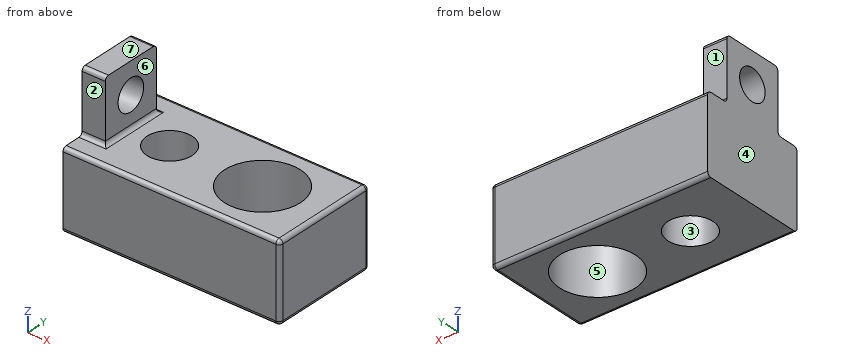
from build123d import *

# Parameters (mm, degrees)
SKETCH1_W           = 14
SKETCH1_H           = 7
BOSS_EXTRUDE1_DEPTH = 5
SKETCH2_R           = 2.45
SKETCH2_R_2         = 1.45
CUT_EXTRUDE1_DEPTH  = 10.287087811
SKETCH5_W           = 4
SKETCH5_H           = 4
BOSS_EXTRUDE3_DEPTH = 1.5
SKETCH9_R           = 1
CUT_EXTRUDE2_DEPTH  = 2
FILLET1_R           = 0.25


with BuildPart() as part:
    # Sketch1 → Boss-Extrude1 (new body)
    with BuildSketch(Plane.XY):
        Rectangle(SKETCH1_W, SKETCH1_H)
    extrude(amount=BOSS_EXTRUDE1_DEPTH)

    # Sketch2 → Cut-Extrude1 (cut, through all)
    with BuildSketch(Plane.XY):
        with Locations((3, 0)):
            Circle(SKETCH2_R)
        with Locations((-3, 0)):
            Circle(SKETCH2_R_2)
    extrude(amount=CUT_EXTRUDE1_DEPTH, mode=Mode.SUBTRACT)

    # Sketch5 → Boss-Extrude3 (add)
    with BuildSketch(Plane.ZY.offset(7)):
        with Locations((7, 0)):
            Rectangle(SKETCH5_W, SKETCH5_H)
    extrude(amount=-BOSS_EXTRUDE3_DEPTH)

    # Sketch9 → Cut-Extrude2 (cut)
    with BuildSketch(Plane(origin=(-5.5, 0, 0), x_dir=(0, 0, -1), z_dir=(1, 0, 0))):
        with Locations((-7, 0)):
            Circle(SKETCH9_R)
    extrude(amount=-CUT_EXTRUDE2_DEPTH, mode=Mode.SUBTRACT)

    # Fillet1
    fillet1_edges = [part.edges().sort_by_distance(p)[0] for p in [
        (7, 0, 5),
        (0, 3.5, 5),
        (-5.5, 0, 5),
        (-6.25, -2, 5),
        (-6.25, 2, 5),
        (-6.25, 2, 9),
        (-6.25, -2, 9),
        (0, 3.5, 0),
        (7, 0, 0),
        (0, -3.5, 0),
        (7, 3.5, 2.5),
        (7, -3.5, 2.5),
        (0, -3.5, 5),
    ]]
    fillet(fillet1_edges, radius=FILLET1_R)


solid = part.part
Can you work these out from the model? Positions are in its coordinate system, mm. Face numbers are marked on the shaded views. A direction names the side the tool comes from. Give positions to 0.01 mm unless a question says otherwise; leave off trailing zeros. Loops run counter-clockwise (first coordinate to the right, second up) from the corner with the lowest first, then second, coordinate; pieces in that order, holes last. Notation, with made-up numbers: M 7,88.5 L 15,88.5 A23 ccw 15,97.5 Z; hole C 51,49 d5. An arc over 180 degrees is marked long. One line per item, written item: value.
1) Imagine slicing it at B-B on x = -3. Write out the boundary of the cut face in (y, z).
Geometry check:
outline: M -3.5,0.25 A0.25 ccw -3.25,0 L -1.45,0 L -1.45,5 L -3.25,5 A0.25 ccw -3.5,4.75 Z; M 1.45,0 L 3.25,0 A0.25 ccw 3.5,0.25 L 3.5,4.75 A0.25 ccw 3.25,5 L 1.45,5 Z
2) On a 3-axis mill with a long thin cutter (end or side, diameter ignored), from which of +Z, -Z, +X, -X, +Y, -Y can I reach the whole of each face in a straight line? I mean the marked faces 1, 2 and 3. Say none if no direction works.
Geometry check:
face 1: +Z, +X, -X, +Y
face 2: +Z, +X, -X, -Y
face 3: +Z, -Z
3) I'm going to push flat-ended pins straight in: pin 1 (2 mm diameter, centred on x = 3.5, y = -2.5, fed in from +Z); pin 2 (1.1 mm diameter, centred on y = -1, z = 6.5, fed in from +X); pin 3 (1.2 mm diameter, centred on x = -6.5, z = 7.5, fed in from -Y); pin 4 (1.5 mm diameter, centred on x = 0.5, y = -0.5, fed in from -Z). Where does each tip first touch, or does it pass through?
Geometry check:
pin 1: stops at z = 5
pin 2: stops at x = -5.5
pin 3: stops at y = -2
pin 4: stops at z = 0
4) Imagine slicing it at D-D on z = 4.5. Write out the boundary of the cut face in (x, y), and give its area (3 significant figures).
Geometry check:
outline: M -7,-3.5 L 6.75,-3.5 A0.25 ccw 7,-3.25 L 7,3.25 A0.25 ccw 6.75,3.5 L -7,3.5 Z; hole C -3,0 d2.9; hole C 3,0 d4.9
area: 72.5 mm²
5) Imagine slicing it at C-C on z = 7. Write out the boundary of the cut face in (x, y), and give its area (3 significant figures).
Geometry check:
outline: M -7,-2 L -5.5,-2 L -5.5,-1 L -7,-1 Z; M -7,1 L -5.5,1 L -5.5,2 L -7,2 Z
area: 3.00 mm²
6) Imagine slicing it at A-A on y = 0. Write out the boundary of the cut face in (x, z), and give its area (3 significant figures).
Geometry check:
outline: M -7,0 L -4.45,0 L -4.45,5 L -5.25,5 A0.25 cw -5.5,5.25 L -5.5,6 L -7,6 Z; M -7,8 L -5.5,8 L -5.5,9 L -7,9 Z; M -1.55,0 L 0.55,0 L 0.55,5 L -1.55,5 Z; M 5.45,0 L 6.75,0 A0.25 ccw 7,0.25 L 7,4.75 A0.25 ccw 6.75,5 L 5.45,5 Z
area: 34.0 mm²
7) Thinking about a two-plate mould opening in X: for the marked faces 4, 5, 6 and 7, which applies, +X half, -X half, draft (parallel to the pull), parting line (faces both ways), or undercut?
Geometry check:
face 4: -X half
face 5: undercut
face 6: +X half
face 7: draft
8) Please list where these lines run through material, in increasing order: line 1 (X direction, y = 0, z = 4.75); line 2 (Y direction, x = -6.55, z = 7); line 3 (Y direction, x = 3, z = 3.5).
Geometry check:
line 1: x = -7 to -4.45, -1.55 to 0.55, 5.45 to 7
line 2: y = -2 to -1, 1 to 2
line 3: y = -3.5 to -2.45, 2.45 to 3.5
